Work out the finished part from the listing and answer in its coordinate system (mm). Give positions to 0.01 mm unless a question says otherwise; leave off trailing zeros. Order: outer loops, then holes, each group sorted by start corner. A loop starts at its lowest first (then second) coordinate and runs counter-clockwise, first axis right, second up. Notation, with made-up numbers: (67.5, 84) - (95.5, 84) arc R19 cw to (95.5, 116) - close; hole circle Ø9 at (-32.75, 71). An arc over 180 degrees is marked (long way). Put each result on its own line as item: value.
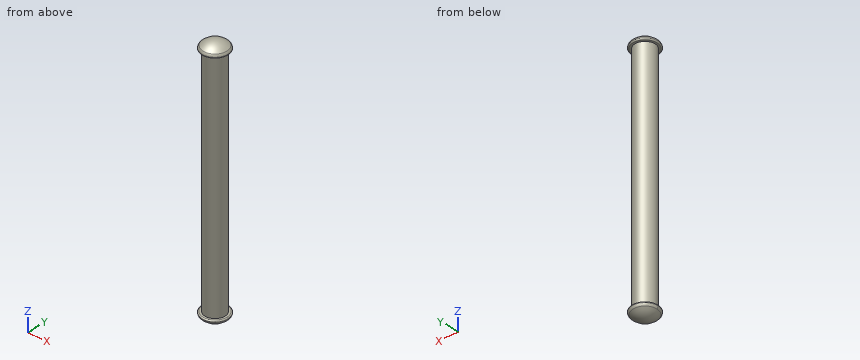
```python
from build123d import *

# Parameters (mm, degrees)
SKETCH1_R                  = 0.5
BOSS_EXTRUDE1_DEPTH        = 5.8
SKETCH2_R                  = 0.65
BOSS_EXTRUDE2_DEPTH        = 0.1
DOME1_FACE_RADIUS          = 0.65
DOME1_HEIGHT               = 0.3
FILLET1_R                  = 0.2
FILLET3_R                  = 0.05
MIRROR2_COPY_1_FACE_RADIUS = 0.65
MIRROR2_COPY_1_HEIGHT      = 0.3
FILLET1_OF_MIRROR2_R       = 0.2
FILLET3_OF_MIRROR2_R       = 0.05


with BuildPart() as part:
    # Sketch1 → Boss-Extrude1 (new, symmetric)
    with BuildSketch(Plane.XY):
        Circle(SKETCH1_R)
    extrude(amount=BOSS_EXTRUDE1_DEPTH, both=True)

    # Sketch2 → Boss-Extrude2 (add)
    with BuildSketch(Plane.XY.offset(5.8)):
        Circle(SKETCH2_R)
    boss_extrude2 = extrude(amount=BOSS_EXTRUDE2_DEPTH)

    # Dome1: a dome of height H over a round flat face of radius A is a cap of a sphere of radius (A * A + H * H) / (2 * H)
    dome1_r = (DOME1_FACE_RADIUS * DOME1_FACE_RADIUS + DOME1_HEIGHT * DOME1_HEIGHT) / (2 * DOME1_HEIGHT)
    dome1_base = Plane((0, 0, 5.9), z_dir=(0, 0, 1))
    with Locations(dome1_base.offset(DOME1_HEIGHT - dome1_r)):
        dome1_ball = Sphere(dome1_r, mode=Mode.PRIVATE)
    add(split(dome1_ball, bisect_by=dome1_base, keep=Keep.TOP, mode=Mode.PRIVATE))

    # Fillet1
    fillet1_edges = [part.edges().sort_by_distance(p)[0] for p in [
        (-0.65, 0, 5.9),
    ]]
    fillet(fillet1_edges, radius=FILLET1_R)

    # Fillet3
    fillet3_edges = [part.edges().sort_by_distance(p)[0] for p in [
        (-0.65, 0, 5.8),
    ]]
    fillet(fillet3_edges, radius=FILLET3_R)

    # Mirror2: Boss-Extrude2 across plane
    add(boss_extrude2.mirror(Plane.XY))

    # Mirror2 copy 1: a dome of height H over a round flat face of radius A is a cap of a sphere of radius (A * A + H * H) / (2 * H)
    mirror2_copy_1_r = (MIRROR2_COPY_1_FACE_RADIUS * MIRROR2_COPY_1_FACE_RADIUS + MIRROR2_COPY_1_HEIGHT * MIRROR2_COPY_1_HEIGHT) / (2 * MIRROR2_COPY_1_HEIGHT)
    mirror2_copy_1_base = Plane((0, 0, -5.9), z_dir=(0, 0, -1))
    with Locations(mirror2_copy_1_base.offset(MIRROR2_COPY_1_HEIGHT - mirror2_copy_1_r)):
        mirror2_copy_1_ball = Sphere(mirror2_copy_1_r, mode=Mode.PRIVATE)
    add(split(mirror2_copy_1_ball, bisect_by=mirror2_copy_1_base, keep=Keep.TOP, mode=Mode.PRIVATE))

    # Fillet1 of Mirror2
    fillet1_of_mirror2_edges = [part.edges().sort_by_distance(p)[0] for p in [
        (-0.65, 0, -5.9),
    ]]
    fillet(fillet1_of_mirror2_edges, radius=FILLET1_OF_MIRROR2_R)

    # Fillet3 of Mirror2
    fillet3_of_mirror2_edges = [part.edges().sort_by_distance(p)[0] for p in [
        (-0.65, 0, -5.8),
    ]]
    fillet(fillet3_of_mirror2_edges, radius=FILLET3_OF_MIRROR2_R)


solid = part.part
```
(1) Straight lines are drawn through the part: line 1 (Y direction, x = 0, z = 4.75); line 2 (Z direction, x = 0.3, y = -0.45). For each, find the intervals that lie inside material, in ascending order.
Geometry check:
line 1: y = -0.5 to 0.5
line 2: z = -6.01 to -5.8, 5.8 to 6.01
(2) Given pin 1 (0.6 mm diameter, centred on x = 0.5, y = 0, fed in from -Z), flat-ended and moving along its own axis, determine where the tip first touches the part or whether it passes through.
Geometry check:
pin 1: stops at z = -6.18
(3) Section A-A, the plane z = 3.25 is taken. Write down the section's boundary in (x, y).
Geometry check:
outline: circle Ø1 at (0, 0)
